Input: part model. Units: mm. Frame: model coordinates. Coordinates: 2 decimals unless noted, no trailing zeros. Order: outer loops, then holes, each group sorted by start corner. A loop starts at its lowest first (then second) coordinate and runs counter-clockwise, first axis right, second up. Notation, with made-up numbers: (39.25, 84) - (43.25, 84) arc R15 cw to (43.25, 103) - close; hole circle Ø6 at (-26.75, 73.5). An arc over 180 degrees is marked (long way). Answer as CSV lines item,"result". Start each with the question number.
Item 1: First-contact query: pin 1 (1 mm diameter, centred on y = 3, z = 22, fed in from -X); pin 2 (4 mm diameter, centred on x = 0, y = 0, fed in from -Z); pin 3 (2 mm diameter, centred on y = -1.5, z = 25.5, fed in from +X). Flat tips, straight axial feed; report the tip coordinate or a pass-through.
Item 2: Material intervals for line 1 along Y through (x, z) = (0, 14.5); line 2 along Y through (x, z) = (-1.5, 9); line 3 along X through (y, z) = (-0.5, 21), sorted ascending.
Item 3: Section A-A (x = 0). Output: boundary loops of the cut face in (y, z), and give its area (3 significant figures).
Item 4: Section D-D (x = -4.5). Output: boundary loops of the cut face in (y, z).
Item 5: Section C-C (y = -1.75). Output: boundary loops of the cut face in (x, z).
Item 6: Section B-B (z = 27.75). Output: boundary loops of the cut face in (x, y).
Item 7: Draft query along X for faces 1 (the flat face through (0, -5, 15)), 2 (the flat face through (-4.31, 2.535, 14.79)), 3 (the cylindrical face through (-0.54, -2.44, 14.79)). Return one class per face: +X half, -X half, draft (parallel to the pull), parting line (faces both ways), or undercut.
from build123d import *

# Parameters (mm, degrees)
BOSS_EXTRUDE1_DEPTH = 30
SKETCH2_R           = 2.5
CUT_EXTRUDE1_DEPTH  = 20


with BuildPart() as part:
    # Sketch1 → Boss-Extrude1 (new body)
    with BuildSketch(Plane.XY):
        Polygon((-5.773502692, 0), (-2.886751346, -5), (2.886751346, -5), (5.773502692, 0), (2.886751346, 5), (-2.886751346, 5), align=None)
    extrude(amount=BOSS_EXTRUDE1_DEPTH)

    # Sketch2 → Cut-Extrude1 (cut)
    with BuildSketch(Plane.XY.offset(30)):
        Circle(SKETCH2_R)
    cut_extrude1 = extrude(amount=-CUT_EXTRUDE1_DEPTH, mode=Mode.SUBTRACT)

    # Mirror1: Cut-Extrude1 across plane
    add(cut_extrude1.mirror(Plane.XY.offset(15)), mode=Mode.SUBTRACT)


solid = part.part
Determined:
1,pin 1,"stops at x = -4.33"
1,pin 2,"passes through"
1,pin 3,"stops at x = 5.48"
2,line 1,"y = -5 to -2.5, 2.5 to 5"
2,line 2,"y = -5 to -2, 2 to 5"
2,line 3,"x = -5.48 to -2.45, 2.45 to 5.48"
3,outline,"(-5, 0) - (-2.5, 0) - (-2.5, 30) - (-5, 30) - close; (2.5, 0) - (5, 0) - (5, 30) - (2.5, 30) - close"
3,area,"150 mm^2"
4,outline,"(-2.21, 0) - (2.21, 0) - (2.21, 30) - (-2.21, 30) - close"
5,outline,"(-4.76, 0) - (-1.79, 0) - (-1.79, 30) - (-4.76, 30) - close; (1.79, 0) - (4.76, 0) - (4.76, 30) - (1.79, 30) - close"
6,outline,"(-5.77, 0) - (-2.89, -5) - (2.89, -5) - (5.77, 0) - (2.89, 5) - (-2.89, 5) - close; hole circle Ø5 at (0, 0)"
7,face 1,"draft"
7,face 2,"-X half"
7,face 3,"undercut"
